CAD build for the part. Positions are in the model's coordinates, mm. A direction names the side the tool comes from. Give positions to 0.01 mm unless a question says otherwise; leave off trailing zeros. Write each loop counter-clockwise with the first axis right and the second up, starting at its lowest first coordinate (ties: lowest second). Pieces come first, ordered by that corner, then holes. Notation, with made-up numbers: (-4, 22.5) - (41, 22.5) arc R20 ccw to (41, 44.5) - close; hole circle Ø10 at (-21.5, -31). An arc over 180 degrees is marked (long way). Answer as a JSON object with one key per item and string values.
from build123d import *

# Parameters (mm, degrees)
HEXAGONSOCKET_DEPTH = 2.2
HEADFILLET_R        = 0.25
CHAMFER_2_SIZE      = 0.5415
SKETCH4_W           = 5
SKETCH4_H           = 5
LPATTERN10_COUNT    = 10
LPATTERN10_PITCH    = 0.6498


with BuildPart() as part:
    # Sketch1 → Base (revolve)
    with BuildSketch(Plane.XY):
        Polygon((0, 0), (0, 6.72), (3.72, 3), (10, 3), (10, 0), align=None)
    revolve(axis=Axis((-0.587069181, 0, 0), (1, 0, 0)))

    # Sketch2 → HexagonSocket (cut)
    with BuildSketch(Plane(origin=(0, 0, 0), x_dir=(0, 0, -1), z_dir=(1, 0, 0))):
        Polygon((2.309401077, 0), (1.154700538, 2), (-1.154700538, 2), (-2.309401077, 0), (-1.154700538, -2), (1.154700538, -2), align=None)
    extrude(amount=HEXAGONSOCKET_DEPTH, mode=Mode.SUBTRACT)

    # Sketch3 → Cut-Revolve1 (revolve, cut)
    with BuildSketch(Plane.XY):
        Polygon((2.2, 2), (3.354700538, 0), (2.2, 0), align=None)
    revolve(axis=Axis((-0.439109555, 0, 0), (1, 0, 0)), mode=Mode.SUBTRACT)

    # HeadFillet
    headfillet_edges = [part.edges().sort_by_distance(p)[0] for p in [
        (3.72, -3, 0),
    ]]
    fillet(headfillet_edges, radius=HEADFILLET_R)

    # Chamfer 2
    chamfer_2_edges = [part.edges().sort_by_distance(p)[0] for p in [
        (10, -3, 0),
    ]]
    chamfer(chamfer_2_edges, length=CHAMFER_2_SIZE)

    # Sketch4 → Cut-Revolve2 (revolve, cut)
    with BuildSketch(Plane(origin=(0, 0, 0), x_dir=(1, 0, 0), z_dir=(0, 1, 0))):
        with Locations((0.5, 8.17)):
            Rectangle(SKETCH4_W, SKETCH4_H)
    revolve(axis=Axis((11.853138686, 0, 0), (-1, 0, 0)), mode=Mode.SUBTRACT)

    # Sketch5 → Cut-Revolve10 (revolve, cut)
    with BuildSketch(Plane.XY):
        Polygon((9.4585, 2.531047244), (9.72925, 3), (9.72925, 3.5415), (9.18775, 3.5415), (9.18775, 3), align=None)
    cut_revolve10 = revolve(axis=Axis((0, 0, 0), (1, 0, 0)), mode=Mode.SUBTRACT)

    # LPattern10: Cut-Revolve10 ×10
    with Locations(*[(-i * LPATTERN10_PITCH, 0, 0) for i in range(1, LPATTERN10_COUNT)]):
        add(cut_revolve10, mode=Mode.SUBTRACT)


solid = part.part
(1) 3-axis set-ups, long thin cutter, end or side, ignore diameter. For faces 3 (the face through (1, -2, 0)), 4 (the face through (10, 0, 0)): which of +Z, -Z, +X, -X, +Y, -Y reach the whole face in a straight line?
Answer key:
{"face 3": "-X", "face 4": "+Z, -Z, +X, +Y, -Y"}
(2) Pull direction X, two halves, no side cores. Call faces 1 (the face through (1.085, -1.014, -1.724)), 2 (the face through (3.34, -1, -3)): pulls with the +X half, pulls with the -X half, needs draft (parallel to the pull), parting line crosses it, or undercut.
Answer key:
{"face 1": "needs draft", "face 2": "pulls with the +X half"}
(3) Flat gauge pins, fed straight in: P1, Ø2, axis at y = 4.5, z = -1.5, coming from the +X side; P2, Ø6, axis at x = 8.5, z = -0.5, coming from the +Y side; P3, Ø0.7, axis at x = 1.5, z = 0, coming from the -Y side. Where does each tip first touch, or does it go through?
Answer key:
{"P1": "stops at x = 2.98", "P2": "stops at y = 3", "P3": "stops at y = -5.57"}
(4) Saw through at A-A, the plane x = 1.5. Give the cut face in (y, z).
Answer key:
{"outline": "circle Ø10.44 at (0, 0); hole (-2, -1.15) - (0, -2.31) - (2, -1.15) - (2, 1.15) - (0, 2.31) - (-2, 1.15) - close"}
(5) Probe L1, parallel to Y at x = 9.5, z = 0.75; L2, parallel to X at y = 3.5, z = -1; L3, parallel to X at y = 0.75, z = 1.75. List the from-to ranges inside material, lowest first. Write a range as [from, to].
Answer key:
{"L1": "y = [-2.49, 2.49]", "L2": "x = [0, 3.08]", "L3": "x = [2.26, 10]"}
